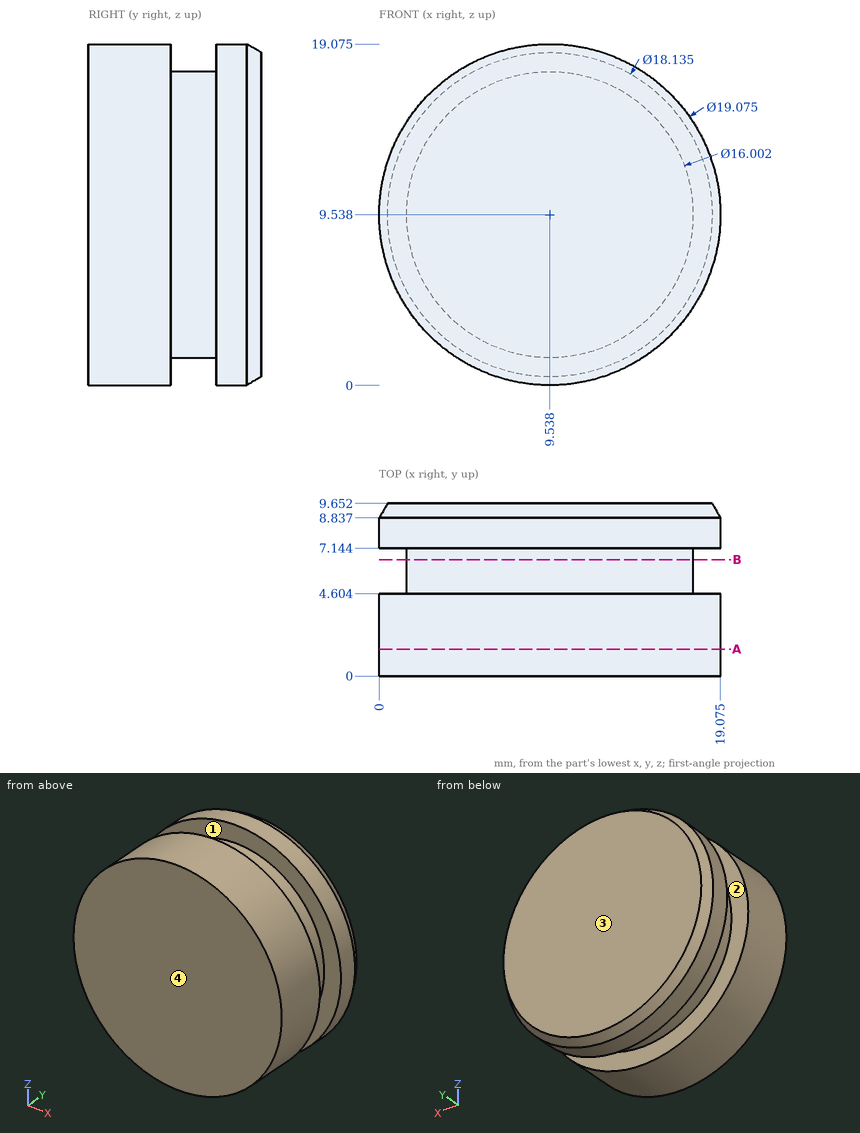
Answer from the drawing. Dimensions are ordinates in mm from the lowest x, y and z of the part. Round coordinates to 2 decimals unless told otherwise and drop trailing zeros. Write each loop counter-clockwise with the first axis right and the second up, starting at its lowest first coordinate (ties: lowest second). Pieces come first, ordered by that corner, then holes. Notation, with made-up numbers: (-13.75, 64) - (24.25, 64) arc R30 ccw to (24.25, 95) - close; hole circle Ø1 at (-34, -39). An arc over 180 degrees is marked (long way). One line per item, written item: value.
Q1. Each of these flat-tipped pins is pushed along its axis until it touches: P1, Ø1, axis at y = 2.5, z = 5.5, coming from the -X side; P2, Ø1.5, axis at y = 7.5, z = 5.5, coming from the -X side (1 decimal). Where does it stop, or does it pass through?
The answers:
P1: stops at x = 0.68
P2: stops at x = 0.6
Q2. Find section A-A (y = 1.5). Determine the outline of the cut face in (x, z) (1 decimal).
The answers:
outline: circle Ø19.1 at (9.5, 9.5)
Q3. Find section B-B (y = 6.5). Determine the outline of the cut face in (x, z), and give its area (3 significant figures).
The answers:
outline: circle Ø16 at (9.54, 9.54)
area: 201 mm2
Q4. For a pull along Y with two mould halves and no side action, classify the marked faces 1, 2, 3 and 4 as pulls with the +Y half, pulls with the -Y half, needs draft (parallel to the pull), parting line crosses it, or undercut.
The answers:
face 1: undercut
face 2: undercut
face 3: pulls with the +Y half
face 4: pulls with the -Y half
Q5. Straight lines are drawn through the part: line 1 (Y direction, x = 2, z = 6.5); line 2 (Z direction, x = 9.25, y = 4.5) (1 decimal); line 3 (X direction, y = 5.25, z = 12.25) (1 decimal). For each, find the intervals that lie inside material, in ascending order. Write a range as from..to.
The answers:
line 1: y = 0..4.6, 7.14..9.65
line 2: z = 0..19.1
line 3: x = 2..17.1
